Here's the drawing with two shaded views (mm, measured from the low corner). I have some questions. A direction names the side the tool comes from. Give positions to 0.01 mm unless a question says otherwise; leave off trailing zeros. Loops run counter-clockwise (first coordinate to the right, second up) from the corner with the lowest first, then second, coordinate; pieces in that order, holes last. Notation, with made-up numbers: (25, -4) -> (60, -4) arc R26 ccw to (60, 29) -> close; hole circle Ø7 at (86, 45). An arc over 180 degrees is marked (long way). Put each result on its own line as item: value.
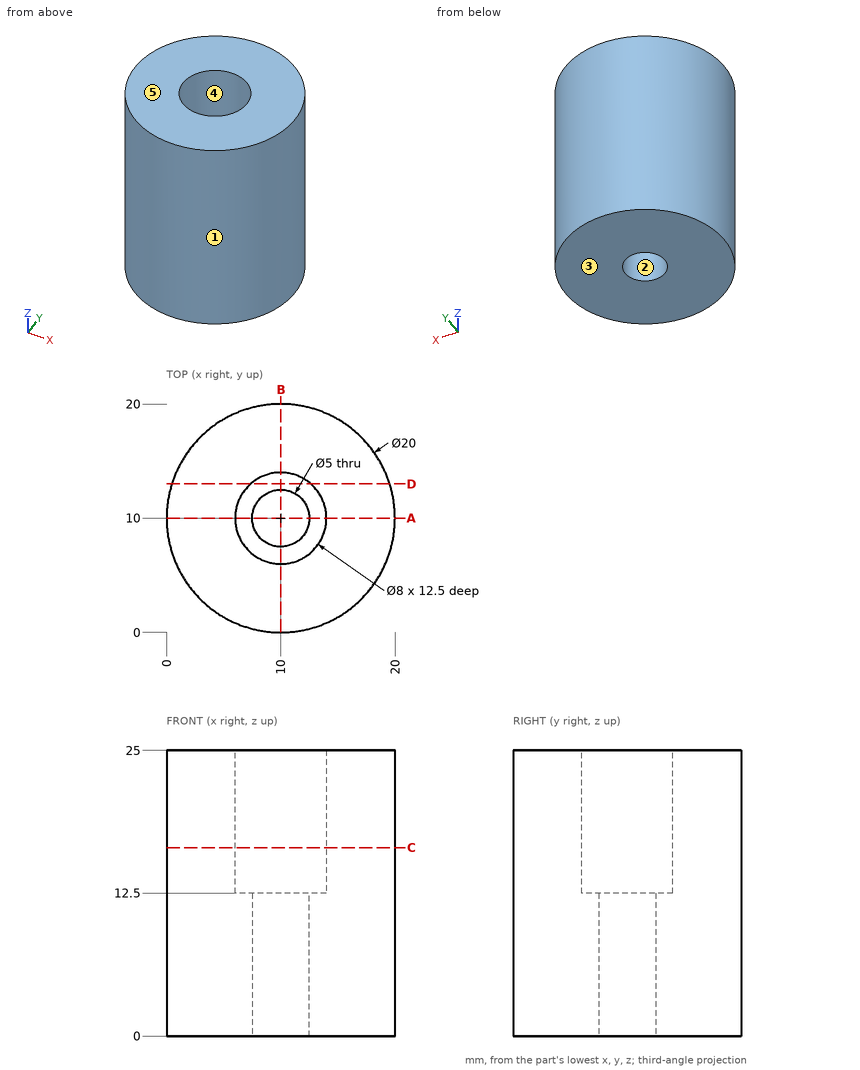
1. If we section it at D-D (y = 13): List the corners of the cut face in (x, z) for me.
Recorded:
outline: (0.46, 0) -> (19.54, 0) -> (19.54, 25) -> (12.65, 25) -> (12.65, 12.5) -> (7.35, 12.5) -> (7.35, 25) -> (0.46, 25) -> close
2. I need wall thicknesses on line 1 (Y direction, x = 10, z = 5.5); line 2 (Y direction, x = 10, z = 18); line 3 (Z direction, x = 8.25, y = 7.75). Which ranges of each line are inside material? Lowest first, please.
Recorded:
line 1: y = 0 to 7.5, 12.5 to 20
line 2: y = 0 to 6, 14 to 20
line 3: z = 0 to 12.5
3. If we section it at A-A (y = 10): List the corners of the cut face in (x, z) for me, then the cut area to 4 significant figures.
Recorded:
outline: (0, 0) -> (7.5, 0) -> (7.5, 12.5) -> (6, 12.5) -> (6, 25) -> (0, 25) -> close; (12.5, 0) -> (20, 0) -> (20, 25) -> (14, 25) -> (14, 12.5) -> (12.5, 12.5) -> close
area: 337.5 mm^2
4. If we section it at C-C (z = 16.5): List the corners of the cut face in (x, y) for me.
Recorded:
outline: circle Ø20 at (10, 10); hole circle Ø8 at (10, 10)
5. Thinking about a two-plate mould opening in X: for the marked faces 1, 2 and 3, which applies, pulls with the +X half, pulls with the -X half, needs draft (parallel to the pull), parting line crosses it, or undercut?
Recorded:
face 1: parting line crosses it
face 2: undercut
face 3: needs draft
6. For the marked faces 4 and 5, which set-ups out of +Z, -Z, +X, -X, +Y, -Y let a thin tool reach every point of the face, with its end or its side?
Recorded:
face 4: +Z
face 5: +Z, +X, -X, +Y, -Y
7. I'm going to push flat-ended pins straight in: pin 1 (5 mm diameter, centred on y = 2.5, z = 18.5, fed in from -X); pin 2 (4 mm diameter, centred on y = 14.5, z = 3.5, fed in from -X); pin 3 (1.5 mm diameter, centred on x = 8.5, z = 21.5, fed in from -Y); pin 4 (4.5 mm diameter, centred on x = 10, y = 10, fed in from +Z). Where does each tip first touch, or does it pass through?
Recorded:
pin 1: stops at x = 1.34
pin 2: stops at x = 0.32
pin 3: stops at y = 0.03
pin 4: passes through
